For this review, use the dimensioned drawing (mm, ordinates from the lowest corner) and the shaded views. A direction names the side the tool comes from. Coordinates: 2 decimals unless noted, no trailing zeros. Loops run counter-clockwise (first coordinate to the right, second up) from the corner with the lowest first, then second, coordinate; pieces in that order, holes last. Notation, with made-up numbers: (44, 47) -> (65, 47) arc R17 ccw to (65, 73) -> close; hole circle Ø9 at (25, 65). An arc over 180 degrees is marked (long way). Answer as a JSON object with one key per item and string values.
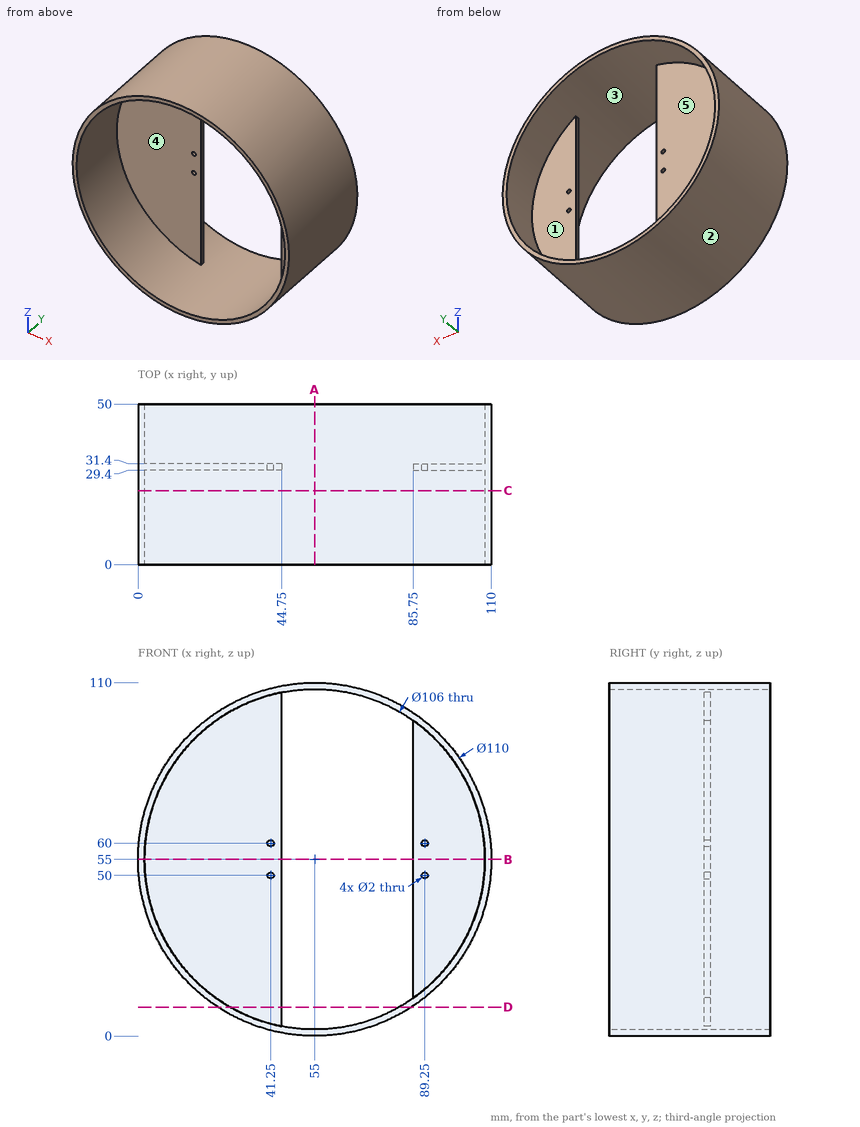
1) For the marked faces 3, 4 and 5, list the 3-axis set-ups (+Z, -Z, +X, -X, +Y, -Y) from which the entire face can be reached by the end or side of a thin tool; tool diameter is ignored.
Completed:
{"face 3": "none", "face 4": "-Y", "face 5": "+Y"}
2) Add section C-C, the plane y = 23. Give the boundary of the cut face in (x, z).
Completed:
{"outline": "circle Ø110 at (55, 55); hole circle Ø106 at (55, 55)"}
3) Add section B-B, the plane z = 55. Give the boundary of the cut face in (x, y), and give its area (3 significant figures).
Completed:
{"outline": "(0, 0) -> (2, 0) -> (2, 29.4) -> (44.75, 29.4) -> (44.75, 31.4) -> (2, 31.4) -> (2, 50) -> (0, 50) -> close; (85.75, 29.4) -> (108, 29.4) -> (108, 0) -> (110, 0) -> (110, 50) -> (108, 50) -> (108, 31.4) -> (85.75, 31.4) -> close", "area": "330 mm²"}
4) Clearance check with flat-ended pins moving along their axes: pin 1 Ø13 at (x, z) = (22.5, 56) entering from -Y; pin 2 Ø1.6 at (x, z) = (89.25, 60) entering from -Y; pin 3 Ø2 at (y, z) = (30, 53.5) entering from +X; pin 4 Ø2 at (y, z) = (31, 53.5) entering from -X. State where each tip first meets the part, or that it passes through.
Completed:
{"pin 1": "y = 29.4", "pin 2": "through", "pin 3": "x = 110", "pin 4": "x = 0"}
5) Add section D-D, the plane z = 9. Give the boundary of the cut face in (x, y), and give its area (3 significant figures).
Completed:
{"outline": "(24.85, 0) -> (28.68, 0) -> (28.68, 29.4) -> (44.75, 29.4) -> (44.75, 31.4) -> (28.68, 31.4) -> (28.68, 50) -> (24.85, 50) -> close; (81.32, 0) -> (85.15, 0) -> (85.15, 50) -> (81.32, 50) -> close", "area": "415 mm²"}
6) Wall thickness on probe 1 along X at (y, z) = (29.85, 60); probe 2 along X at (y, z) = (39, 55); probe 3 along Y at (x, z) = (40, 20.5): over which ranges is each line inside the solid? List them lowest first.
Completed:
{"probe 1": "0.23 to 40.25, 42.25 to 44.75, 85.75 to 88.25, 90.25 to 109.77", "probe 2": "0 to 2, 108 to 110", "probe 3": "29.4 to 31.4"}
7) Add section A-A, the plane x = 55. Give the boundary of the cut face in (y, z), and give its area (3 significant figures).
Completed:
{"outline": "(0, 0) -> (50, 0) -> (50, 2) -> (0, 2) -> close; (0, 108) -> (50, 108) -> (50, 110) -> (0, 110) -> close", "area": "200 mm²"}
8) The part is to be moulded in two halves that separate along Z. For the marked faces 1 and 2, say which applies: pulls with the +Z half, pulls with the -Z half, needs draft (parallel to the pull), parting line crosses it, or undercut.
Completed:
{"face 1": "undercut", "face 2": "parting line crosses it"}
